from build123d import *

# Parameters (mm, degrees)
SKETCH1_W            = 140
SKETCH1_H            = 70
BOSS_EXTRUDE1_DEPTH  = 5
SKETCH2_W            = 130
SKETCH2_H            = 60
BOSS_EXTRUDE2_DEPTH  = 5
M3_CLEARANCE_HOLE1_D = 3


with BuildPart() as part:
    # Sketch1 → Boss-Extrude1 (new body)
    with BuildSketch(Plane.XY):
        with Locations((70, 35)):
            Rectangle(SKETCH1_W, SKETCH1_H)
    extrude(amount=BOSS_EXTRUDE1_DEPTH)

    # Sketch2 → Boss-Extrude2 (add)
    with BuildSketch(Plane.XY.offset(5)):
        with Locations((70, 35)):
            Rectangle(SKETCH2_W, SKETCH2_H)
    extrude(amount=BOSS_EXTRUDE2_DEPTH)

    # M3 Clearance Hole1 (through all)
    with Locations(Plane(origin=(137.5, 2.5, 0), x_dir=(-1, 0, 0), z_dir=(0, 0, -1))):
        with Locations((0, 0), (0, 65), (135, 0), (135, 65)):
            Hole(M3_CLEARANCE_HOLE1_D / 2)


solid = part.part
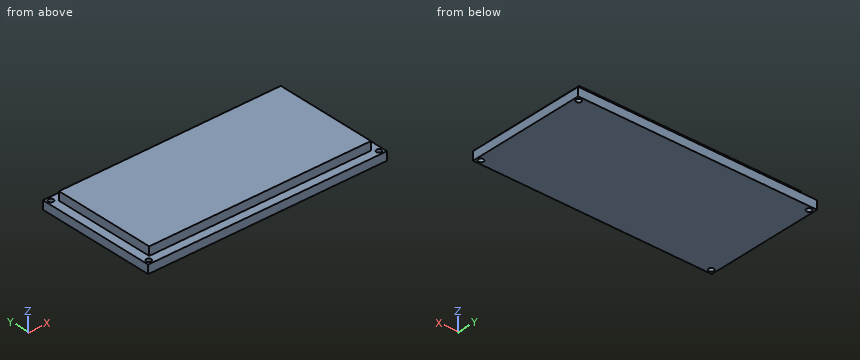
Verification items for the finished model (mm, model axes). Give positions to 0.01 mm unless a question says otherwise; leave off trailing zeros. Write each loop counter-clockwise with the first axis right and the second up, starting at its lowest first coordinate (ties: lowest second). Pieces come first, ordered by that corner, then holes. Notation, with made-up numbers: M 87,-18.75 L 124,-18.75 A20 cw 124,20.25 Z; hole C 6,56.5 d6. An arc over 180 degrees is marked long. Use CSV: the item, a comma, the result in double quotes.
1) Cross-section at D-D (x = 44.5). Enter the section's corners in (y, z).
Final values:
outline,"M 0,0 L 70,0 L 70,5 L 65,5 L 65,10 L 5,10 L 5,5 L 0,5 Z"
2) Material ranges on line 1 along Y through (x, z) = (137.5, 2.2); line 2 along X through (y, z) = (67.5, 1.15); line 3 along X through (y, z) = (6.5, 6.75), recorded low to high.
Final values:
line 1,"0 to 1, 4 to 66, 69 to 70"
line 2,"0 to 1, 4 to 136, 139 to 140"
line 3,"5 to 135"
3) Cross-section at B-B (y = 67.5). Enter the section's corners in (x, z), plus the area to 3 significant figures.
Final values:
outline,"M 0,0 L 1,0 L 1,5 L 0,5 Z; M 4,0 L 136,0 L 136,5 L 4,5 Z; M 139,0 L 140,0 L 140,5 L 139,5 Z"
area,"670 mm²"
4) Cross-section at A-A (x = 2.5). Enter the section's corners in (y, z).
Final values:
outline,"M 0,0 L 1,0 L 1,5 L 0,5 Z; M 4,0 L 66,0 L 66,5 L 4,5 Z; M 69,0 L 70,0 L 70,5 L 69,5 Z"
5) Go/stop test with flat-tipped pins: pin 1 Ø5 at (x, y) = (2.5, 2.5) entering from +Z; pin 2 Ø2.5 at (y, z) = (35, 8.5) entering from +X; pin 3 Ø4 at (x, z) = (73.5, 7.5) entering from +Y. Record where each tip stops, or that it passes through.
Final values:
pin 1,"z = 5"
pin 2,"x = 135"
pin 3,"y = 65"
6) Cross-section at C-C (y = 23). Enter the section's corners in (x, z), plus the area to 3 significant figures.
Final values:
outline,"M 0,0 L 140,0 L 140,5 L 135,5 L 135,10 L 5,10 L 5,5 L 0,5 Z"
area,"1,350 mm²"
